from build123d import *

# Parameters (mm, degrees)
SKETCH_1_R          = 11
SKETCH_1_R_2        = 2.5
EXTRUDE_1_DEPTH     = 3
SKETCH_2_R          = 1.5
CUT_EXTRUDE_2_DEPTH = 439.330925215
SKETCH_3_W          = 50
SKETCH_3_H          = 20
CUT_EXTRUDE_3_DEPTH = 439.330925215
FILLET_1_R          = 3


with BuildPart() as part:
    # 草图1 → 凸台-拉伸1 (new body)
    with BuildSketch(Plane(origin=(0, 0, 0), x_dir=(1, 0, 0), z_dir=(0, 1, 0))):
        with BuildLine():
            Line((0, 0), (71.32346865, 85))
            Line((71.32346865, 85), (358.67653135, 85))
            Line((358.67653135, 85), (430, 0))
            Line((430, 0), (336.457513111, 0))
            ThreePointArc((336.457513111, 0), (310, -10), (283.542486889, 0))
            Line((283.542486889, 0), (146.457513111, 0))
            ThreePointArc((146.457513111, 0), (120, -10), (93.542486889, 0))
            Line((93.542486889, 0), (0, 0))
        make_face()
        with Locations(Location((120, 30, 0), (0, 0, 270))):
            Circle(SKETCH_1_R, mode=Mode.SUBTRACT)
        with Locations(Location((310, 30, 0), (0, 0, 90))):
            Circle(SKETCH_1_R, mode=Mode.SUBTRACT)
        with Locations(Location((106, 30, 0), (0, 0, 270))):
            Circle(SKETCH_1_R_2, mode=Mode.SUBTRACT)
        with Locations(Location((134, 30, 0), (0, 0, 270))):
            Circle(SKETCH_1_R_2, mode=Mode.SUBTRACT)
        with Locations(Location((324, 30, 0), (0, 0, 90))):
            Circle(SKETCH_1_R_2, mode=Mode.SUBTRACT)
        with Locations(Location((296, 30, 0), (0, 0, 90))):
            Circle(SKETCH_1_R_2, mode=Mode.SUBTRACT)
    extrude(amount=EXTRUDE_1_DEPTH)

    # 草图2 → 切除-拉伸2 (cut, through all)
    with BuildSketch(Plane(origin=(0, 3, 0), x_dir=(1, 0, 0), z_dir=(0, 1, 0))):
        with Locations(Location((221, 13.5, 0), (0, 0, 270))):
            Circle(SKETCH_2_R)
        with Locations(Location((304, 13.5, 0), (0, 0, 270))):
            Circle(SKETCH_2_R)
        with Locations(Location((316, 13.5, 0), (0, 0, 270))):
            Circle(SKETCH_2_R)
        with Locations(Location((388.5, 13.5, 0), (0, 0, 270))):
            Circle(SKETCH_2_R)
        with Locations(Location((400.5, 13.5, 0), (0, 0, 270))):
            Circle(SKETCH_2_R)
        with Locations(Location((366, 9, 0), (0, 0, 270))):
            Circle(SKETCH_2_R)
        with Locations(Location((366, 21, 0), (0, 0, 270))):
            Circle(SKETCH_2_R)
        with Locations(Location((221, 81, 0), (0, 0, 270))):
            Circle(SKETCH_2_R)
        with Locations(Location((333.5, 81, 0), (0, 0, 270))):
            Circle(SKETCH_2_R)
        with Locations(Location((345.5, 81, 0), (0, 0, 270))):
            Circle(SKETCH_2_R)
        with Locations(Location((358.183504016, 79.364671789, 0), (0, 0, 270))):
            Circle(SKETCH_2_R)
        with Locations(Location((365.896955332, 70.172138471, 0), (0, 0, 270))):
            Circle(SKETCH_2_R)
        with Locations(Location((408.320937572, 19.613205225, 0), (0, 0, 270))):
            Circle(SKETCH_2_R)
        with Locations(Location((416.034388888, 10.420671908, 0), (0, 0, 270))):
            Circle(SKETCH_2_R)
        with Locations(Location((209, 81, 0), (0, 0, 90))):
            Circle(SKETCH_2_R)
        with Locations(Location((96.5, 81, 0), (0, 0, 90))):
            Circle(SKETCH_2_R)
        with Locations(Location((84.5, 81, 0), (0, 0, 90))):
            Circle(SKETCH_2_R)
        with Locations(Location((71.816495984, 79.364671789, 0), (0, 0, 90))):
            Circle(SKETCH_2_R)
        with Locations(Location((64.103044668, 70.172138471, 0), (0, 0, 90))):
            Circle(SKETCH_2_R)
        with Locations(Location((21.679062428, 19.613205225, 0), (0, 0, 90))):
            Circle(SKETCH_2_R)
        with Locations(Location((13.965611112, 10.420671908, 0), (0, 0, 90))):
            Circle(SKETCH_2_R)
        with Locations(Location((29.5, 13.5, 0), (0, 0, 90))):
            Circle(SKETCH_2_R)
        with Locations(Location((41.5, 13.5, 0), (0, 0, 90))):
            Circle(SKETCH_2_R)
        with Locations(Location((64, 21, 0), (0, 0, 90))):
            Circle(SKETCH_2_R)
        with Locations(Location((64, 9, 0), (0, 0, 90))):
            Circle(SKETCH_2_R)
        with Locations(Location((114, 13.5, 0), (0, 0, 90))):
            Circle(SKETCH_2_R)
        with Locations(Location((126, 13.5, 0), (0, 0, 90))):
            Circle(SKETCH_2_R)
        with Locations(Location((209, 13.5, 0), (0, 0, 90))):
            Circle(SKETCH_2_R)
    extrude(amount=-CUT_EXTRUDE_2_DEPTH, mode=Mode.SUBTRACT)

    # 草图3 → 切除-拉伸3 (cut, through all)
    with BuildSketch(Plane(origin=(0, 3, 0), x_dir=(1, 0, 0), z_dir=(0, 1, 0))):
        with Locations((215, 35)):
            Rectangle(SKETCH_3_W, SKETCH_3_H)
    extrude(amount=-CUT_EXTRUDE_3_DEPTH, mode=Mode.SUBTRACT)

    # 圆角1
    fillet_1_edges = [part.edges().sort_by_distance(p)[0] for p in [
        (190, 1.5, -25),
        (190, 1.5, -45),
        (240, 1.5, -45),
        (240, 1.5, -25),
    ]]
    fillet(fillet_1_edges, radius=FILLET_1_R)


solid = part.part
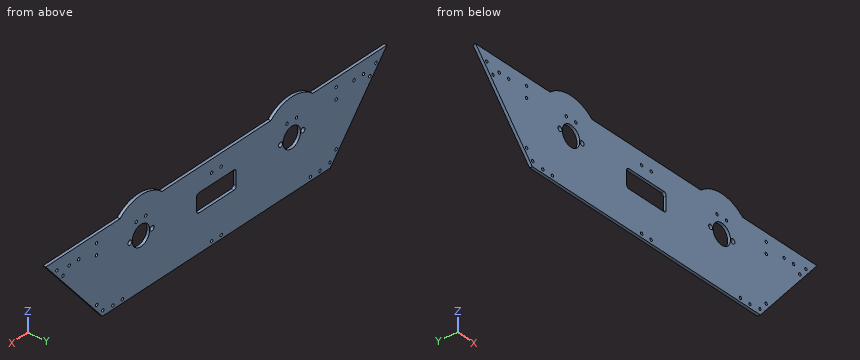
Part model, mm, in its own coordinate system. Round coordinates to 2 decimals unless told otherwise and drop trailing zeros. Order: outer loops, then holes, each group sorted by start corner. A loop starts at its lowest first (then second) coordinate and runs counter-clockwise, first axis right, second up. Notation, with made-up numbers: (-17.5, 4.25) -> (25.5, 4.25) arc R19 cw to (25.5, 15.25) -> close; hole circle Ø7 at (-17, 49.5). An arc over 180 degrees is marked (long way). Put each result on its own line as item: value.
Q1. Band-saw the part on C-C (y = 2.15). State how many separate pieces and enclosed holes the cut face has, and give its area (3 significant figures).
From the geometry:
separate pieces: 1
enclosed holes: 35
area: 29,200 mm2
Q2. Wall check: line 1 (Z direction, x = 221, y = 1.2); line 2 (Z direction, x = 218.5, y = 2.4); line 3 (X direction, y = 1.8, z = -69). Give the ranges that are in metal, low to high. Write a range as [from, to].
From the geometry:
line 1: z = [-85, -82.5], [-79.5, -45], [-25, -15], [-12, 0]
line 2: z = [-85, -45], [-25, 0]
line 3: x = [57.9, 63.17], [65.04, 364.96], [366.83, 372.1]
Q3. Band-saw the part on D-D (z = -54). Give the cut face in (x, y).
From the geometry:
outline: (45.31, 0) -> (384.69, 0) -> (384.69, 3) -> (45.31, 3) -> close
Q4. Band-saw the part on A-A (x = 120). Give the cut face in (y, z), and give its area (3 significant figures).
From the geometry:
outline: (0, -85) -> (3, -85) -> (3, -41) -> (0, -41) -> close; (0, -19) -> (3, -19) -> (3, 10) -> (0, 10) -> close
area: 219 mm2
Q5. Pin check, flat tips, straight feed: pin 1 Ø1 at (y, z) = (2.5, -65) entering from -X; pin 2 Ø0.9 at (x, y) = (232, 1) entering from +Z; pin 3 Ø1 at (x, y) = (141.5, 0.5) entering from +Z. Stop position of each tip, or through.
From the geometry:
pin 1: stops at x = 54.12
pin 2: stops at z = 0
pin 3: stops at z = 4.04
Q6. Band-saw the part on B-B (z = -37). Give the cut face in (x, y), and give its area (3 significant figures).
From the geometry:
outline: (31.05, 0) -> (111.51, 0) -> (111.51, 3) -> (31.05, 3) -> close; (128.49, 0) -> (190, 0) -> (190, 3) -> (128.49, 3) -> close; (240, 0) -> (301.51, 0) -> (301.51, 3) -> (240, 3) -> close; (318.49, 0) -> (398.95, 0) -> (398.95, 3) -> (318.49, 3) -> close
area: 852 mm2
